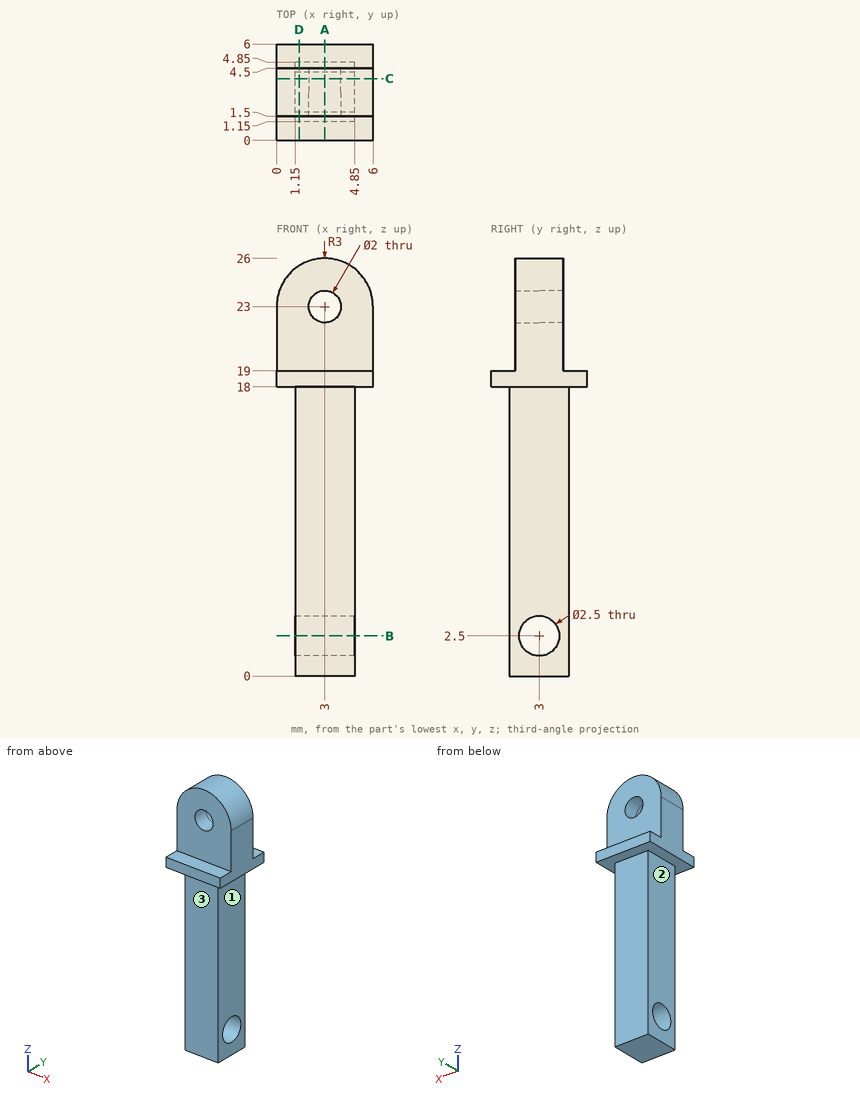
Part print with two shaded views. Sizes in mm from the minimum x, y, z corner. A direction names the side the tool comes from. Give positions to 0.01 mm unless a question says otherwise; leave off trailing zeros. Order: outer loops, then holes, each group sorted by start corner. A loop starts at its lowest first (then second) coordinate and runs counter-clockwise, first axis right, second up.
(1) Saw through at B-B, the plane z = 2.5. Give the cut face in (x, y).
(2) Saw through at C-C, the plane y = 3.85. Give the cut face in (x, z).
(3) Saw through at D-D, the plane x = 1.4. Give the cut face in (y, z).
(4) Saw through at A-A, the plane x = 3. Give the cut face in (y, z), then the cut area to 3 significant figures.
(5) Tool access for the marked faces 1, 2 and 3: list every direction of +Z, -Z, +X, -X, +Y, -Y with a clear straight run to the whole face (end or side of a thin tool).
(6) Drill centre lines: L1, parallel to X at y = 3.65, z = 23; L2, parallel to Z at x = 3, y = 1.95; L3, parallel to Z at x = 3, y = 2.45. Where is each one in solid material? Low to high.
(7) Flat gauge pins, fed straight in: pin 1 (1.8 mm diameter, centred on y = 3.5, z = 8.5, fed in from -X); pin 2 (3 mm diameter, centred on x = 2.5, z = 23.5, fed in from +Y); pin 3 (1.5 mm diameter, centred on x = 2.5, z = 3, fed in from -Y). Where does each tip first touch, or does it go through?
Results found:
1. outline: (1.15, 1.15) - (4.85, 1.15) - (4.85, 1.75) - (1.15, 1.75) - close; (1.15, 4.25) - (4.85, 4.25) - (4.85, 4.85) - (1.15, 4.85) - close
2. outline: (0, 18) - (1.15, 18) - (1.15, 3.42) - (4.85, 3.42) - (4.85, 18) - (6, 18) - (6, 23) arc R3 ccw to (0, 23) - close; (1.15, 0) - (4.85, 0) - (4.85, 1.58) - (1.15, 1.58) - close; hole circle Ø2 at (3, 23)
3. outline: (0, 18) - (1.15, 18) - (1.15, 0) - (4.85, 0) - (4.85, 18) - (6, 18) - (6, 19) - (4.5, 19) - (4.5, 25.54) - (1.5, 25.54) - (1.5, 19) - (0, 19) - close; hole circle Ø2.5 at (3, 2.5)
4. outline: (0, 18) - (1.15, 18) - (1.15, 0) - (4.85, 0) - (4.85, 18) - (6, 18) - (6, 19) - (4.5, 19) - (4.5, 22) - (1.5, 22) - (1.5, 19) - (0, 19) - close; (1.5, 24) - (4.5, 24) - (4.5, 26) - (1.5, 26) - close; hole circle Ø2.5 at (3, 2.5)
4. area: 82.7 mm2
5. face 1: -Z, +X, +Y, -Y
5. face 2: -Z, -X, +Y, -Y
5. face 3: -Z, +X, -X, -Y
6. L1: x = 0 to 2, 4 to 6
6. L2: z = 0 to 1.82, 3.18 to 22, 24 to 26
6. L3: z = 0 to 1.38, 3.62 to 22, 24 to 26
7. pin 1: stops at x = 1.15
7. pin 2: stops at y = 4.5
7. pin 3: stops at y = 1.15
